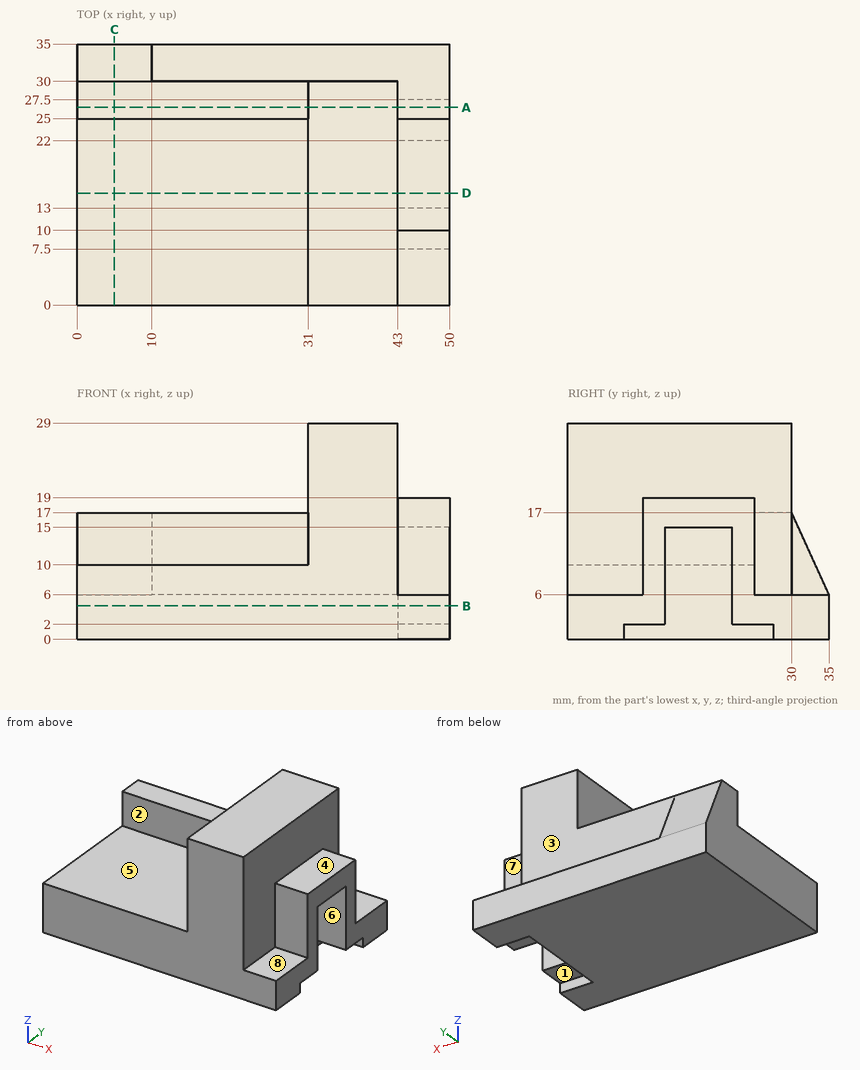
Verification items for this drawing (mm, ordinates from the low corner). A direction names the side the tool comes from. Give positions to 0.01 mm unless a question says otherwise; leave off trailing zeros. Write each loop counter-clockwise with the first axis right and the second up, starting at its lowest first coordinate (ties: lowest second). Pieces come first, ordered by that corner, then holes. Notation, with made-up numbers: (-7, 6.5) - (28, 6.5) arc R7 ccw to (28, 17.5) - close; hole circle Ø5 at (44.5, -30). An arc over 180 degrees is marked (long way). Answer as a JSON object with one key per item and string values. Group by question number.
1) Sectioned sample at D-D (y = 15). Record the cut outline in (x, z).
2) Access from +Z, -Z, +X, -X, +Y, -Y to the whole of each face (thin tool, end or side, straight path). Record for the marked faces 5, 6, 7 and 8.
3) Thickness scan on probe 1 along Y at (x, z) = (47, 9); probe 2 along Y at (x, z) = (44, 3.25); probe 3 along Z at (x, y) = (14.5, 22.5). Record the ranges inside material, lowest first. Write a range as from..to.
4) Sectioned sample at A-A (y = 26.5). Record the cut outline in (x, z), then the cut area to 3 significant figures.
5) Sectioned sample at C-C (x = 5). Record the cut outline in (y, z).
6) Release check for a two-part mould opening along Y. For the marked faces 1, 2, 3 and 4 record: pulls with the +Y half, pulls with the -Y half, needs draft (parallel to the pull), parting line crosses it, or undercut.
7) Sectioned sample at B-B (z = 4.5). Record the cut outline in (x, y).
8) Depth check by flat-ended pin: P1, Ø3, axis at y = 4.5, z = 8, coming from the +X side; P2, Ø11.5, axis at x = 25, z = 14.5, coming from the +Y side; P3, Ø1.6, axis at x = 47, y = 24.5, coming from the -Z side. Enter the tip coordinate at first touch or a pass-through.
Geometry results:
{
 "1": {"outline": "(0, 0) - (43, 0) - (43, 15) - (50, 15) - (50, 19) - (43, 19) - (43, 29) - (31, 29) - (31, 10) - (0, 10) - close"},
 "2": {"face 5": "+Z, -X, -Y", "face 6": "-Z, +X", "face 7": "+Z, +X, +Y", "face 8": "+Z, +X, -Y"},
 "3": {"probe 1": "y = 10..13, 22..25", "probe 2": "y = 0..13, 22..35", "probe 3": "z = 0..10"},
 "4": {"outline": "(0, 0) - (43, 0) - (43, 2) - (50, 2) - (50, 6) - (43, 6) - (43, 29) - (31, 29) - (31, 17) - (0, 17) - close", "area": "903 mm^2"},
 "5": {"outline": "(0, 0) - (35, 0) - (35, 6) - (30, 17) - (25, 17) - (25, 10) - (0, 10) - close"},
 "6": {"face 1": "undercut", "face 2": "pulls with the -Y half", "face 3": "pulls with the +Y half", "face 4": "needs draft"},
 "7": {"outline": "(0, 0) - (50, 0) - (50, 13) - (43, 13) - (43, 22) - (50, 22) - (50, 35) - (0, 35) - close"},
 "8": {"P1": "stops at x = 43", "P2": "stops at y = 30", "P3": "stops at z = 2"}
}
